Source: three-view drawing plus pictorial views. Frame: mm from the lowest corner of the part. A direction names the side the tool comes from. Give positions to 0.01 mm unless a question says otherwise; leave off trailing zeros. Loops run counter-clockwise (first coordinate to the right, second up) from the corner with the lowest first, then second, coordinate; pieces in that order, holes last. Notation, with made-up numbers: (74, 20.25) - (79, 20.25) arc R21 ccw to (79, 36.25) - close; hole circle Ø9 at (45.25, -22). An arc over 180 degrees is marked (long way). Answer as a JSON object with one key per item and string values. Group by question number.
(1) Section query C-C (x = 12). Return loops of the section in (y, z) (1 decimal), plus the area to 3 significant figures.
(2) Mould query, pull axis X, two halves, no side actions, for the marked faces 1 and 2. Classes: +X half, -X half, draft (parallel to the pull), parting line (faces both ways), or undercut.
(3) Access query for the marked faces 3, 4, 5 and 6. Directions: +Z, -Z, +X, -X, +Y, -Y. A direction counts if a zero-diameter tool reaches every point of the face in a straight line with its end or side. Return the directions, or none.
(4) Section query B-B (y = 1.75). Count the separate pieces of the cut face and the enclosed holes in it, plus the area to 3 significant figures.
(5) Section query A-A (x = 38.1). Return loops of the section in (y, z) (1 decimal).
(6) Material intervals for L1, parallel to Z at x = 38.1, y = 0.7; L2, parallel to X at y = 1.3, z = 11 (1 decimal); L3, parallel to X at y = 1, z = 11.75, sorted ascending.
(7) Pin query (flat end, axial travel): P1, Ø1.6, axis at y = 2, z = 1.5, coming from the +X side; P2, Ø1, axis at x = 13.5, y = 2.5, coming from the +Z side; P3, Ø1.6, axis at x = 40, y = 1.5, coming from the -Z side. Return the tip coordinate at first contact, or that it passes through.
(8) Section query D-D (x = 5.5). Return loops of the section in (y, z) (1 decimal).
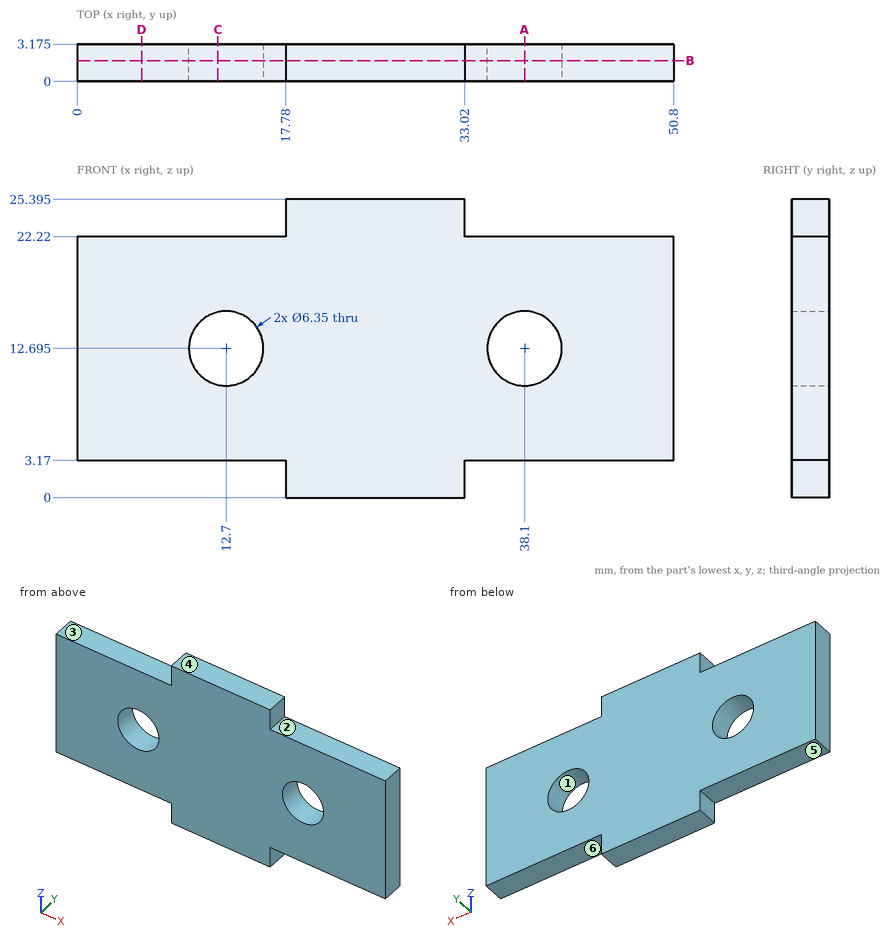
Recorded:
{
 "1": {"outline": "(0, 3.2) - (3.2, 3.2) - (3.2, 9.6) - (0, 9.6) - close; (0, 15.8) - (3.2, 15.8) - (3.2, 22.2) - (0, 22.2) - close", "area": "40.8 mm^2"},
 "2": {"face 1": "undercut", "face 2": "draft"},
 "3": {"face 3": "+Z, -X, +Y, -Y", "face 4": "+Z, +X, -X, +Y, -Y", "face 5": "-Z, -X, +Y, -Y", "face 6": "-Z, +X, +Y, -Y"},
 "4": {"separate pieces": "1", "enclosed holes": "2", "area": "1,000 mm^2"},
 "5": {"outline": "(0, 3.2) - (3.2, 3.2) - (3.2, 9.5) - (0, 9.5) - close; (0, 15.9) - (3.2, 15.9) - (3.2, 22.2) - (0, 22.2) - close"},
 "6": {"L1": "z = 3.17 to 9.52, 15.87 to 22.22", "L2": "x = 0 to 10, 15.4 to 35.4, 40.8 to 50.8", "L3": "x = 0 to 9.67, 15.73 to 35.07, 41.13 to 50.8"},
 "7": {"P1": "stops at x = 33.02", "P2": "stops at z = 22.22", "P3": "stops at z = 3.17"},
 "8": {"outline": "(0, 3.2) - (3.2, 3.2) - (3.2, 22.2) - (0, 22.2) - close"}
}
